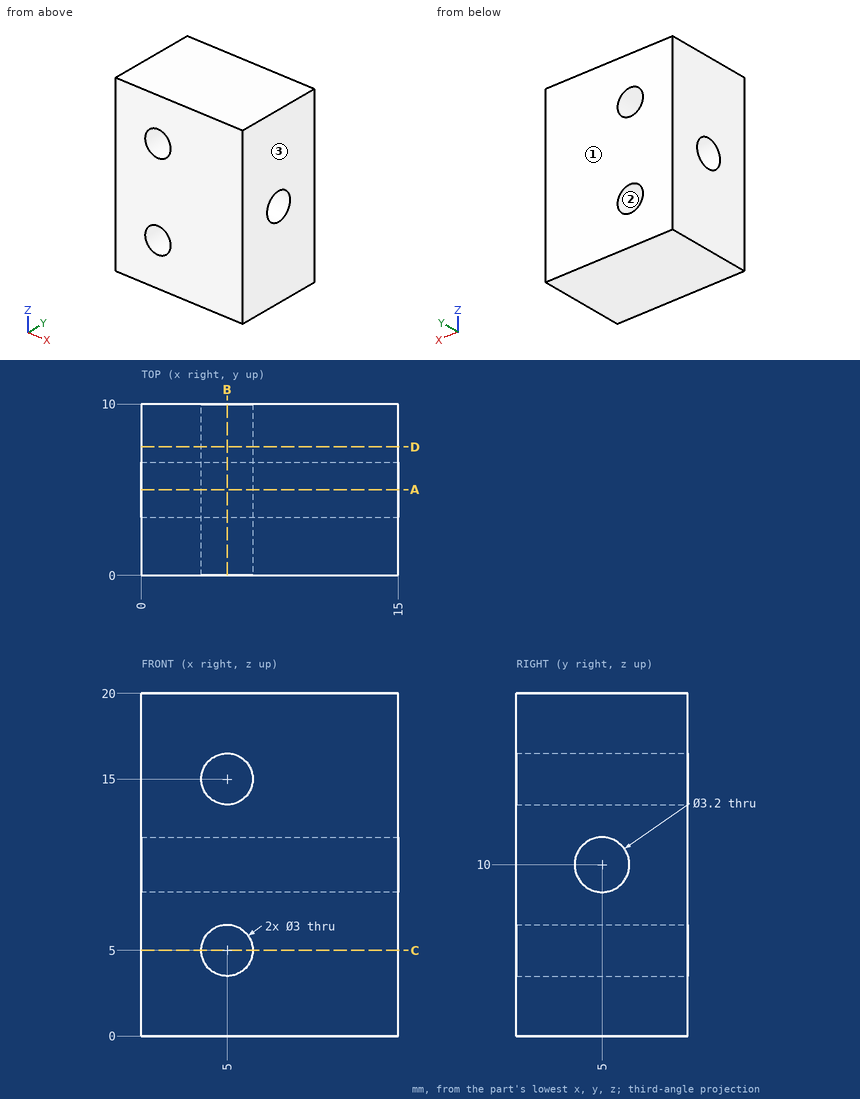
Can you work these out from the drawing? Everything is in mm from the part's minimum corner. Give positions to 0.01 mm unless a question says otherwise; leave off trailing zeros. Loops run counter-clockwise (first coordinate to the right, second up) from the corner with the lowest first, then second, coordinate; pieces in that order, holes last. Notation, with made-up numbers: M 39.25,-30 L 90.25,-30 A26 cw 90.25,3 Z; hole C -12.75,47.25 d11. An arc over 180 degrees is marked long. Use CSV: the item, a comma, the result in double quotes. Start each with the question number.
1. Imagine slicing it at A-A, the plane y = 5. Write out the boundary of the cut face in (x, z), plus the area to 3 significant figures.
2. Imagine slicing it at D-D, the plane y = 7.5. Write out the boundary of the cut face in (x, z).
3. For P1, Ø3, axis at y = 5, z = 10, coming from the +X side, with a flat end and sliding along its axis, tell me the tip position at first contact or that it passes through.
4. If we mould it in two halves opening along X, with no side actions, what happens to the marked faces 1, 2 and 3? For each: released by +X, released by -X, zero draft, split by the parting line, or undercut.
5. If I drill on L1, parallel to Z at x = 5, y = 7.5; L2, parallel to Y at x = 4.5, z = 10; L3, parallel to Z at x = 5.5, y = 3, over which ranges is the centre line in solid material (lowest first)?
6. Imagine slicing it at C-C, the plane z = 5. Write out the boundary of the cut face in (x, y), plus the area to 3 significant figures.
7. Imagine slicing it at B-B, the plane x = 5. Write out the boundary of the cut face in (y, z).
Response values:
1,outline,"M 0,0 L 15,0 L 15,8.4 L 0,8.4 Z; M 0,11.6 L 15,11.6 L 15,20 L 0,20 Z; hole C 5,5 d3; hole C 5,15 d3"
1,area,"238 mm^2"
2,outline,"M 0,0 L 15,0 L 15,20 L 0,20 Z; hole C 5,5 d3; hole C 5,15 d3"
3,P1,"through"
4,face 1,"zero draft"
4,face 2,"undercut"
4,face 3,"released by +X"
5,L1,"0 to 3.5, 6.5 to 13.5, 16.5 to 20"
5,L2,"0 to 3.4, 6.6 to 10"
5,L3,"0 to 3.59, 6.41 to 13.59, 16.41 to 20"
6,outline,"M 0,0 L 3.5,0 L 3.5,10 L 0,10 Z; M 6.5,0 L 15,0 L 15,10 L 6.5,10 Z"
6,area,"120 mm^2"
7,outline,"M 0,0 L 10,0 L 10,3.5 L 0,3.5 Z; M 0,6.5 L 10,6.5 L 10,13.5 L 0,13.5 Z; M 0,16.5 L 10,16.5 L 10,20 L 0,20 Z; hole C 5,10 d3.2"
